CAD build for the part. Positions are in the model's coordinates, mm. Face numbers are marked on the shaded views. A direction names the side the tool comes from. Give positions to 0.01 mm unless a question says otherwise; leave off trailing zeros. Write each loop counter-clockwise with the first axis right and the second up, starting at its lowest first coordinate (ties: lowest second). Pieces come first, ordered by that corner, then holes. Notation, with made-up numbers: (63, 56) - (117, 56) arc R21 ccw to (117, 70) - close; hole circle Ø1 at (50.25, 71.5). An arc over 180 degrees is marked (long way). Put each result on its own line as item: value. Start each with the question number.
1. Drop flat-ended pins along their axis: pin 1 (3 mm diameter, centred on x = 16.5, y = -4, fed in from -Z); pin 2 (0.8 mm diameter, centred on y = 1, z = -3, fed in from -X); pin 3 (1.5 mm diameter, centred on x = 10, y = -3.5, fed in from +Z). Give the stop position or say it passes through.
2. Tool access for the marked faces 1 and 2: list every direction of +Z, -Z, +X, -X, +Y, -Y with a clear straight run to the whole face (end or side of a thin tool).
3. Cut at C-C on y = -2. List the corners of the cut face in (x, z).
4. Cut at D-D on z = 17. List the corners of the cut face in (x, y).
5. Cut at A-A on z = 9.5. List the corners of the cut face in (x, y), and give its area (3 significant figures).
6. Cut at B-B on x = 7.75. List the corners of the cut face in (y, z).
7. Wall check: line 1 (Z direction, x = 2, y = -0.8); line 2 (Y direction, x = 17.5, z = 4.5); line 3 (Y direction, x = 10, z = 7.75). Give the ranges that are in metal, low to high.
from build123d import *

# Parameters (mm, degrees)
F0_W      = 25
F0_H      = 24
F1_DEPTH  = 1.5
F2_R      = 1
F3_DEPTH  = 1.501
F4_W      = 8
F4_H      = 8
F4_R      = 2.5
F5_DEPTH  = 2
F5_FACE_R = 2.5
F6_DEPTH  = 4
F8_DEPTH  = 1.5


with BuildPart() as f1:
    # F0 (on Front) → F1 (new body)
    with BuildSketch(Plane.XZ):
        with Locations((12.5, 12)):
            Rectangle(F0_W, F0_H)
    extrude(amount=F1_DEPTH)

    # F2 (on face) → F3 (cut, through all)
    with BuildSketch(Plane.XZ.offset(1.5)):
        with Locations((2, 22)):
            Circle(F2_R)
        with Locations((2, 9.5)):
            Circle(F2_R)
        with Locations((23, 22)):
            Circle(F2_R)
        with Locations((23, 9.5)):
            Circle(F2_R)
    extrude(amount=-F3_DEPTH, mode=Mode.SUBTRACT)

    # F4 (on face) → F5 (join)
    with BuildSketch(Plane.XZ.offset(1.5)):
        with Locations((12.5, 9.5)):
            Rectangle(F4_W, F4_H)
        with Locations((12.5, 9.5)):
            Circle(F4_R, mode=Mode.SUBTRACT)
    extrude(amount=F5_DEPTH)

    # F5_face (on face) → F6 (join)
    with BuildSketch(Plane(origin=(12.5, -1.5, 9.5), x_dir=(1, 0, 0), z_dir=(0, -1, 0))):
        Circle(F5_FACE_R)
    extrude(amount=F6_DEPTH)

    # F7 (on face) → F8 (join)
    with BuildSketch(Plane(origin=(0, 0, 0), x_dir=(-1, 0, 0), z_dir=(0, 1, 0))):
        Polygon((-2, 0), (-2, 5), (-23, 5), (-23, 0), (-20.5, 0), (-20.5, -5), (-4.5, -5), (-4.5, 0), align=None)
    extrude(amount=F8_DEPTH)


solid = f1.part
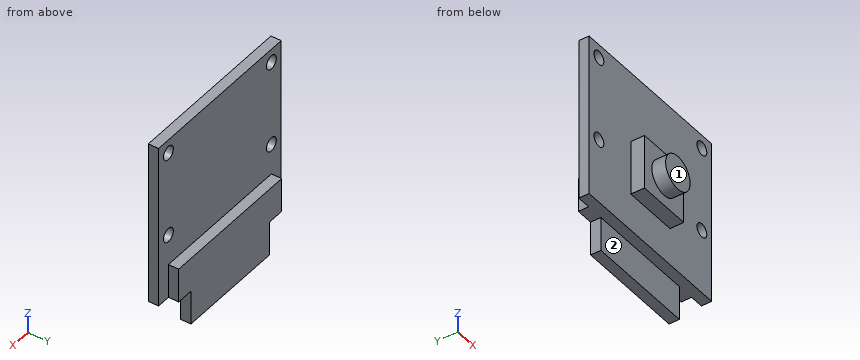
Report:
1. pin 1: stops at z = 5.5
1. pin 2: stops at x = 4.5
1. pin 3: stops at z = 13.5
2. face 1: +Z, -Z, +X, -X, -Y
2. face 2: -Z, +X, -X, -Y
3. outline: (8.5, 5.5) - (16.5, 5.5) - (16.5, 13.5) - (8.5, 13.5) - close
4. outline: (0, -1.5) - (25, -1.5) - (25, 0) - (0, 0) - close
5. outline: (0, -1.5) - (1, -1.5) - (1, 0) - (0, 0) - close; (3, -1.5) - (8.5, -1.5) - (8.5, -3.5) - (10, -3.5) - (10, -5.5) - (15, -5.5) - (15, -3.5) - (16.5, -3.5) - (16.5, -1.5) - (22, -1.5) - (22, 0) - (3, 0) - close; (24, -1.5) - (25, -1.5) - (25, 0) - (24, 0) - close
5. area: 57.5 mm²
6. outline: (-1.5, 0) - (0, 0) - (0, -5) - (1.5, -5) - (1.5, 5) - (0, 5) - (0, 24) - (-1.5, 24) - close
7. line 1: z = 0 to 8.5, 10.5 to 21, 23 to 24
7. line 2: y = -1.5 to 1.5
7. line 3: y = -3.5 to 0
